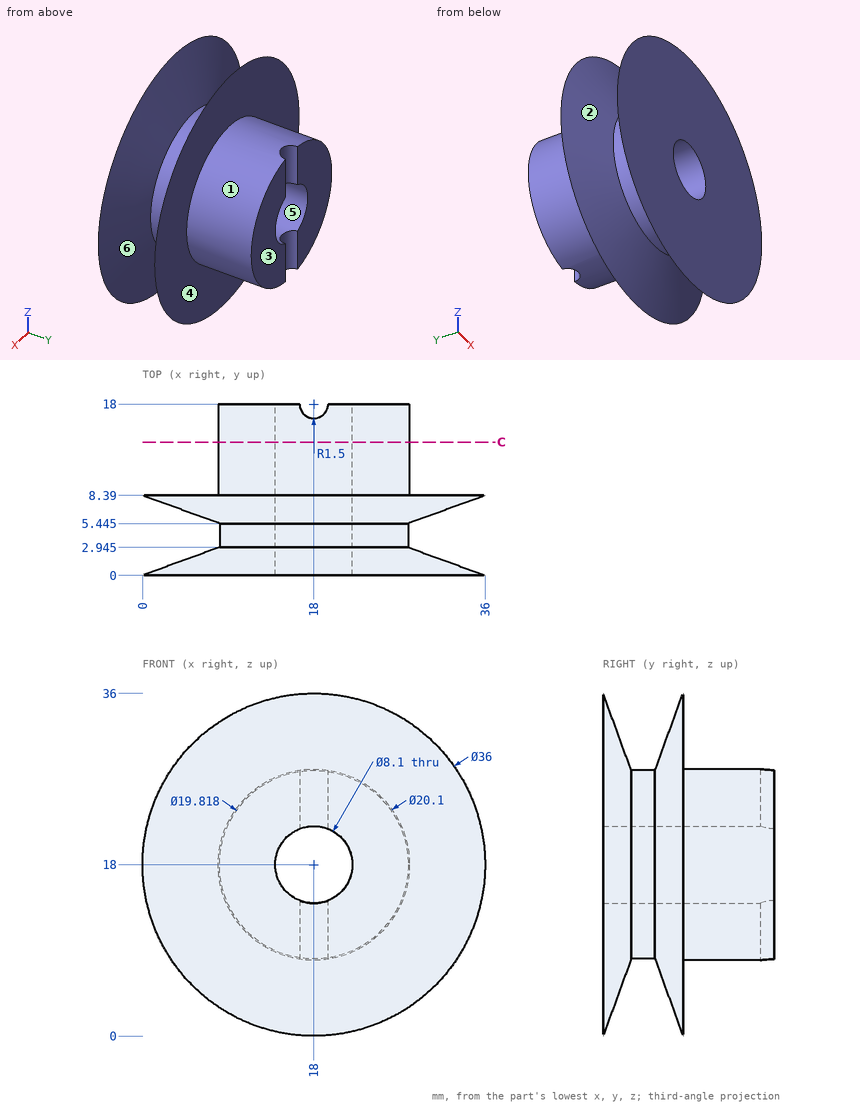
The figure shows three views and two pictorial views of one solid part (mm, origin at its lowest corner). Answer the questions. A direction names the side the tool comes from. Coordinates: 2 decimals unless noted, no trailing zeros. Loops run counter-clockwise (first coordinate to the right, second up) from the corner with the lowest first, then second, coordinate; pieces in that order, holes last. Notation, with made-up numbers: (-30, 84.5) -> (16, 84.5) arc R15 cw to (16, 110.5) -> close; hole circle Ø2 at (-36, 75). An arc over 180 degrees is marked (long way). Write item = value, one per line. Start each with the question number.
1) Given pin 1 Ø10 at (y, z) = (13.5, 12.5) entering from -X; pin 2 Ø5 at (x, z) = (18, 18) entering from -Y; pin 3 Ø18 at (x, z) = (19, 26) entering from +Y; pin 4 Ø1.5 at (x, y) = (18, 4.5) entering from +Z, each flat-ended and moving along its own axis, determine where each tip first touches the part or whether it passes through.
2) A cutting plane is placed at C-C (y = 14). Give the vertices of the cut face in (x, z).
3) Straight lines are drawn through the part: line 1 (X direction, y = 9, z = 18); line 2 (X direction, y = 4.75, z = 18). For each, find the intervals that lie inside material, in ascending order. Write a range as from..to.
4) The mould has two halves that part along Y. Classify the marked faces 4, 5 and 6: released by +Y, released by -Y, zero draft, split by the parting line, or undercut.
5) A tool of negligible diameter and unlimited length cuts with its end or side. For the marked faces 1, 2 and 3, from which of +Z, -Z, +X, -X, +Y, -Y can it reach the whole face along a straight path? Write none if from no direction.
Responses:
q1.pin_1 = 7.96
q1.pin_2 = through
q1.pin_3 = 18
q1.pin_4 = 27.91
q2.outline = circle Ø20.1 at (18, 18); hole circle Ø8.1 at (18, 18)
q3.line_1 = 7.95..13.95, 22.05..28.05
q3.line_2 = 8.09..13.95, 22.05..27.91
q4.face_4 = released by +Y
q4.face_5 = zero draft
q4.face_6 = undercut
q5.face_1 = +Y
q5.face_2 = none
q5.face_3 = +Z, -Z, +X, -X, +Y
